from build123d import *

# Parameters (mm, degrees)
F0_R     = 5.5
F1_DEPTH = 2
F2_R     = 3.5
F3_DEPTH = 5
F4_R     = 4.5
F5_DEPTH = 3
F6_R     = 1.5
F7_DEPTH = 8


with BuildPart() as f1:
    # F0 (on Top) → F1 (new body)
    with BuildSketch(Plane.XY):
        Circle(F0_R)
    extrude(amount=F1_DEPTH)

    # F2 (on face) → F3 (join)
    with BuildSketch(Plane.XY.offset(2)):
        with Locations((0, -1)):
            Circle(F2_R)
    extrude(amount=F3_DEPTH)

    # F4 (on face) → F5 (join)
    with BuildSketch(Plane.XY.offset(7)):
        Circle(F4_R)
    extrude(amount=F5_DEPTH)

    # F6 (on face) → F7 (cut)
    with BuildSketch(Plane(origin=(0, 0, 0), x_dir=(1, 0, 0), z_dir=(0, 0, -1))):
        Circle(F6_R)
    extrude(amount=-F7_DEPTH, mode=Mode.SUBTRACT)


solid = f1.part
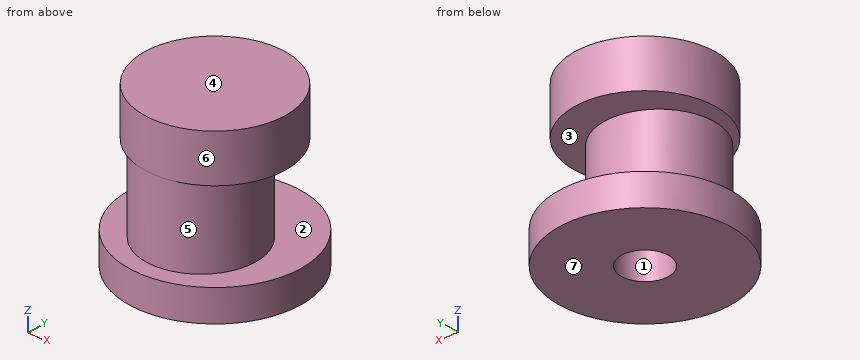
Source: CAD feature listing. Evaluate the final solid. Frame: model axes, mm. Face numbers are marked on the shaded views. A direction names the side the tool comes from. Coordinates: 2 decimals unless noted, no trailing zeros. Loops run counter-clockwise (first coordinate to the right, second up) from the corner with the lowest first, then second, coordinate; pieces in that order, holes last. Notation, with made-up numbers: (-8.5, 0.25) - (-0.5, 0.25) arc R24 cw to (-0.5, 18.25) - close; hole circle Ø4 at (3.5, 60). An arc over 180 degrees is marked (long way). Return JSON: item names as keys, results as strings.
Q1. Material intervals for line 1 along Y through (x, z) = (0, 6.25); line 2 along Z through (x, y) = (-0.75, 2.75); line 3 along Z through (x, y) = (-5, 1.25), sorted ascending.
Results:
{"line 1": "-4.5 to -1.5, 1.5 to 2.5", "line 2": "0 to 2, 7 to 10", "line 3": "0 to 2"}
Q2. Mould query, pull axis Z, two halves, no side actions, for the marked faces 1, 2, 3 and 4. Classes: released by +Z, released by -Z, zero draft, split by the parting line, or undercut.
Results:
{"face 1": "zero draft", "face 2": "undercut", "face 3": "undercut", "face 4": "released by +Z"}
Q3. Section D-D, the plane y = -1. Return loops of the section in (x, z), plus the area to 3 significant figures.
Results:
{"outline": "(-5.41, 0) - (-1.12, 0) - (-1.12, 8) - (1.12, 8) - (1.12, 0) - (5.41, 0) - (5.41, 2) - (3.5, 2) - (3.5, 7) - (4.39, 7) - (4.39, 10) - (-4.39, 10) - (-4.39, 7) - (-3.5, 7) - (-3.5, 2) - (-5.41, 2) - close", "area": "65.1 mm2"}
Q4. Contact query for flat-ended pins moving along their axis: P1, Ø1.5, axis at x = 1, z = 6, coming from the +Y side; P2, Ø1.5, axis at y = 2, z = 7, coming from the -X side. Output: stop coordinate, or through.
Results:
{"P1": "y = 2.49", "P2": "x = -4.32"}
Q5. Section A-A, the plane y = 4. Return loops of the section in (x, z).
Results:
{"outline": "(-3.77, 0) - (3.77, 0) - (3.77, 2) - (-3.77, 2) - close; (-2.06, 7) - (2.06, 7) - (2.06, 10) - (-2.06, 10) - close"}
Q6. Access query for the marked faces 5, 6 and 7. Directions: +Z, -Z, +X, -X, +Y, -Y. A direction counts if a zero-diameter tool reaches every point of the face in a straight line with its end or side. Return the directions, or none.
Results:
{"face 5": "none", "face 6": "+Z", "face 7": "-Z, +X, -X, +Y, -Y"}
Q7. Section C-C, the plane z = 1. Return loops of the section in (x, y), plus the area to 3 significant figures.
Results:
{"outline": "circle Ø11 at (0, 0); hole circle Ø3 at (0, 0)", "area": "88.0 mm2"}
